```python
from build123d import *

# Parameters (mm, degrees)
SKETCH1_R           = 51.054
SKETCH1_R_2         = 49.53
BOSS_EXTRUDE1_DEPTH = 762
SKETCH2_R           = 1.524
CUT_EXTRUDE1_DEPTH  = 66.04
CIRPATTERN1_COUNT   = 6


with BuildPart() as part:
    # Sketch1 → Boss-Extrude1 (new body)
    with BuildSketch(Plane(origin=(0, 0, 0), x_dir=(1, 0, 0), z_dir=(0, 1, 0))):
        with Locations(Location((0, 0, 0), (0, 0, 270))):
            Circle(SKETCH1_R)
        with Locations(Location((0, 0, 0), (0, 0, 270))):
            Circle(SKETCH1_R_2, mode=Mode.SUBTRACT)
    extrude(amount=BOSS_EXTRUDE1_DEPTH)

    # Sketch2 → Cut-Extrude1 (cut)
    with BuildSketch(Plane.XY):
        with Locations(Location((0, 692.15, 0), (0, 0, 90))):
            Circle(SKETCH2_R)
    cut_extrude1 = extrude(amount=-CUT_EXTRUDE1_DEPTH, mode=Mode.SUBTRACT)

    # CirPattern1: Cut-Extrude1 ×6 about axis
    cirpattern1_axis = Axis((0, 762, 0), (0, -1, 0))
    for i in range(1, CIRPATTERN1_COUNT):
        add(cut_extrude1.rotate(cirpattern1_axis, i * 360 / CIRPATTERN1_COUNT), mode=Mode.SUBTRACT)


solid = part.part
```
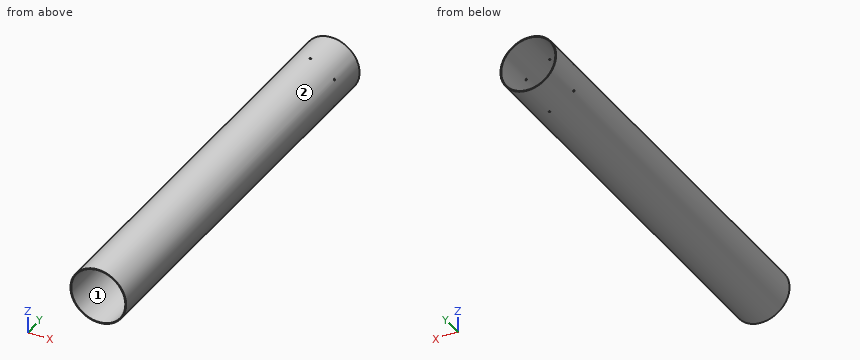
Work out the finished part from the listing and answer in its coordinate system (mm). Face numbers are marked on the shaded views. Round coordinates to 2 decimals unless told otherwise and drop trailing zeros. Write each loop counter-clockwise with the first axis right and the second up, starting at its lowest first coordinate (ties: lowest second). Pieces come first, ordered by that corner, then holes. Notation, with made-up numbers: (29.5, 87.25) - (47.5, 87.25) arc R25 cw to (47.5, 116.25) - close; hole circle Ø5 at (0.25, -25.5). An arc over 180 degrees is marked (long way). Return JSON: item names as keys, results as strings. Group by question number.
Q1. The part is cut by section C-C on x = -28.5. Write down the section's boundary in (y, z), then the cut area to 3 significant figures.
Q2. The part is cut by section B-B on y = 198. Write down the section's boundary in (x, z).
Q3. Find the intervals of material crossed by L1, parallel to X at y = 596, z = 3; L2, parallel to X at y = 325.5, z = 0; L3, parallel to Z at x = -3.5, y = 443, in increasing order.
Q4. The mould has two halves that part along X. Classify the marked faces 1 and 2: released by +X, released by -X, zero draft, split by the parting line, or undercut.
Q5. Each of these flat-tipped pins is pushed along its axis until it touches: pin 1 Ø5 at (y, z) = (127.5, -6.5) entering from -X; pin 2 Ø6 at (y, z) = (232, 0) entering from -X; pin 3 Ø5 at (x, z) = (-30, -34) entering from -Y; pin 4 Ø1.5 at (x, y) = (29, 137.5) entering from -Z. Where does it stop, or does it pass through?
Q6. The part is cut by section A-A on z = 0. Write down the section's boundary in (x, y).
Solved:
{
 "1": {"outline": "(0, -42.36) - (762, -42.36) - (762, -40.51) - (0, -40.51) - close; (0, 40.51) - (762, 40.51) - (762, 42.36) - (0, 42.36) - close", "area": "2,820 mm²"},
 "2": {"outline": "circle Ø102.11 at (0, 0); hole circle Ø99.06 at (0, 0)"},
 "3": {"L1": "-50.97 to -49.44, 49.44 to 50.97", "L2": "-51.05 to -49.53, 49.53 to 51.05", "L3": "-50.93 to -49.41, 49.41 to 50.93"},
 "4": {"face 1": "undercut", "face 2": "split by the parting line"},
 "5": {"pin 1": "x = -50.9", "pin 2": "x = -51.05", "pin 3": "through", "pin 4": "z = -42.53"},
 "6": {"outline": "(-51.05, 0) - (-49.53, 0) - (-49.53, 762) - (-51.05, 762) - close; (49.53, 0) - (51.05, 0) - (51.05, 762) - (49.53, 762) - close"}
}
